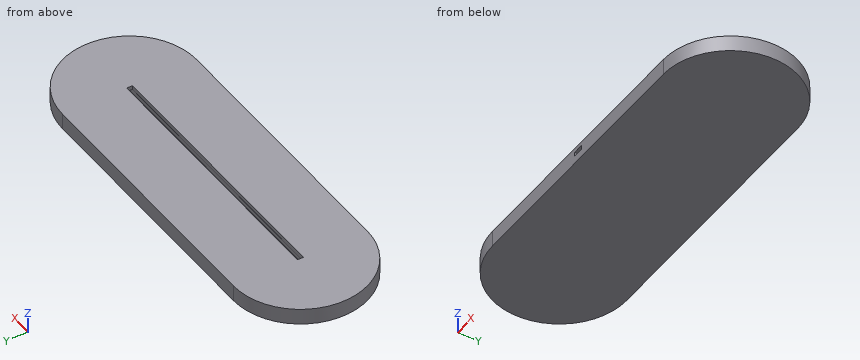
```python
from build123d import *

# Parameters (mm, degrees)
PAD_DEPTH       = 3
PAD001_DEPTH    = 3
SKETCH002_W     = 209.08447
SKETCH002_H     = 4.18
PAD002_DEPTH    = 3
SKETCH003_W     = 26.3
SKETCH003_H     = 34.2
POCKET_DEPTH    = 3
SKETCH004_W     = 18
SKETCH004_H     = 25
POCKET001_DEPTH = 3
SKETCH005_W     = 14
SKETCH005_H     = 5
POCKET002_DEPTH = 6
SKETCH006_W     = 14
SKETCH006_H     = 3
POCKET003_DEPTH = 3
SKETCH007_W     = 8
SKETCH007_H     = 3
POCKET004_DEPTH = 3
SKETCH008_W     = 200
SKETCH008_H     = 4.4
PAD003_DEPTH    = 3


with BuildPart() as part:
    # Sketch → Pad (new body)
    with BuildSketch(Plane.XY):
        with BuildLine():
            ThreePointArc((-100, 50), (-150, 0), (-100, -50))
            Line((-100, -50), (100, -50))
            ThreePointArc((100, -50), (150, 0), (100, 50))
            Line((-100, 50), (100, 50))
        make_face()
    extrude(amount=PAD_DEPTH)

    # Sketch001 (on Face6 of Pad) → Pad001 (join)
    with BuildSketch(Plane.XY.offset(3)):
        with BuildLine():
            ThreePointArc((-100, 50), (-150, 0), (-100, -50))
            Line((-100, -50), (100, -50))
            ThreePointArc((100, -50), (150, 0), (100, 50))
            Line((-100, 50), (100, 50))
        make_face()
        with BuildLine():
            ThreePointArc((-100, 5), (-105, 0), (-100, -5))
            Line((-100, -5), (100, -5))
            ThreePointArc((100, -5), (105, 0), (100, 5))
            Line((-100, 5), (100, 5))
        make_face(mode=Mode.SUBTRACT)
    extrude(amount=PAD001_DEPTH)

    # Sketch002 (on Face9 of Pad001) → Pad002 (join)
    with BuildSketch(Plane.XY.offset(6)):
        with BuildLine():
            ThreePointArc((-100, 50), (-150, 0), (-100, -50))
            Line((-100, -50), (100, -50))
            ThreePointArc((100, -50), (150, 0), (100, 50))
            Line((-100, 50), (100, 50))
        make_face()
        Rectangle(SKETCH002_W, SKETCH002_H, mode=Mode.SUBTRACT)
    extrude(amount=PAD002_DEPTH)

    # Sketch003 (on Face13 of Pad002) → Pocket (cut)
    with BuildSketch(Plane.XY.offset(9)):
        with Locations((0, -29.9)):
            Rectangle(SKETCH003_W, SKETCH003_H)
    extrude(amount=-POCKET_DEPTH, mode=Mode.SUBTRACT)

    # Sketch004 (on Face27 of Pocket) → Pocket001 (cut)
    with BuildSketch(Plane.XY.offset(6)):
        with Locations((0, -25.3)):
            Rectangle(SKETCH004_W, SKETCH004_H)
    extrude(amount=-POCKET001_DEPTH, mode=Mode.SUBTRACT)

    # Sketch005 (on Face13 of Pocket001) → Pocket002 (cut)
    with BuildSketch(Plane.XY.offset(9)):
        with Locations((0, -10.3)):
            Rectangle(SKETCH005_W, SKETCH005_H)
    extrude(amount=-POCKET002_DEPTH, mode=Mode.SUBTRACT)

    # Sketch006 (on Face23 of Pocket002) → Pocket003 (cut)
    with BuildSketch(Plane.XZ.offset(7.8)):
        with Locations((0, 4.5)):
            Rectangle(SKETCH006_W, SKETCH006_H)
    extrude(amount=-POCKET003_DEPTH, mode=Mode.SUBTRACT)

    # Sketch007 (on Face13 of Pocket003) → Pocket004 (cut)
    with BuildSketch(Plane.XY.offset(9)):
        with Locations((0, -48.5)):
            Rectangle(SKETCH007_W, SKETCH007_H)
    extrude(amount=-POCKET004_DEPTH, mode=Mode.SUBTRACT)

    # Sketch008 (on Face15 of Pocket004) → Pad003 (join)
    with BuildSketch(Plane.XY.offset(9)):
        with BuildLine():
            ThreePointArc((-100, 50), (-150, 0), (-100, -50))
            Line((-100, -50), (100, -50))
            ThreePointArc((100, -50), (150, 0), (100, 50))
            Line((-100, 50), (100, 50))
        make_face()
        Rectangle(SKETCH008_W, SKETCH008_H, mode=Mode.SUBTRACT)
    extrude(amount=PAD003_DEPTH)


solid = part.part
```
Geometry: final body of the model. Coordinates: model frame, mm. Give positions to 0.01 mm unless a question says otherwise; leave off trailing zeros. Order: outer loops, then holes, each group sorted by start corner. A loop starts at its lowest first (then second) coordinate and runs counter-clockwise, first axis right, second up. Notation, with made-up numbers: (39, 69) -> (52, 69) arc R24 ccw to (52, 99) -> close; hole circle Ø6 at (10.25, 32). An arc over 180 degrees is marked (long way). Write each question's results on one line, items separated by ' | '. Start each with the question number.
1) Line query: line 1 (Y direction, x = -32, z = 8.25); line 2 (Y direction, x = -68.5, z = 3.25); line 3 (Z direction, x = -5.5, y = -19.5). Output: solid intervals per line, ascending. Write a range as from..to.
2) First-contact query: pin 1 (3.5 mm diameter, centred on y = 0, z = 10, fed in from +X); pin 2 (1.8 mm diameter, centred on y = -10, z = 7.5, fed in from +X); pin 3 (0.9 mm diameter, centred on y = 0, z = 7, fed in from -X). Flat tips, straight axial feed; report the tip coordinate or a pass-through.
3) Section B-B (y = 25). Return loops of the section in (x, z), then the cut area to 3 significant figures.
4) Section A-A (x = 51). Return loops of the section in (y, z), then the cut area to 3 significant figures.
Calculated:
1) line 1: -50..-2.09, 2.09..50 | line 2: -50..-5, 5..50 | line 3: 0..3, 9..12
2) pin 1: x = 150 | pin 2: x = 149.16 | pin 3: x = -150
3) outline: (-143.3, 0) -> (143.3, 0) -> (143.3, 12) -> (-143.3, 12) -> close | area: 3,440 mm2
4) outline: (-50, 0) -> (50, 0) -> (50, 12) -> (2.2, 12) -> (2.2, 9) -> (2.09, 9) -> (2.09, 6) -> (5, 6) -> (5, 3) -> (-5, 3) -> (-5, 6) -> (-2.09, 6) -> (-2.09, 9) -> (-2.2, 9) -> (-2.2, 12) -> (-50, 12) -> close | area: 1,140 mm2
